Could you check a few things on this model? Use its own coordinates, in mm. A direction names the side the tool comes from. Coordinates: 2 decimals unless noted, no trailing zeros. Write each loop counter-clockwise with the first axis right and the second up, starting at its lowest first coordinate (ties: lowest second). Pieces come first, ordered by that corner, then holes.
```python
from build123d import *

# Parameters (mm, degrees)
EXTRUDE_1_DEPTH         = 3
SKETCH_2_W              = 1.5
SKETCH_2_H              = 5
CUT_EXTRUDE_1_DEPTH     = 154.658257181
SKETCH_3_W              = 54.5
SKETCH_3_H              = 3
EXTRUDE_2_DEPTH         = 40
HOLE_WIZARD_2_5_2_5_1_D = 2.5
HOLE_WIZARD_2_5_2_5_2_D = 2.5
HOLE_WIZARD_M641_D      = 71.5
FILLET_1_R              = 0.5
FILLET_2_R              = 3
FILLET_3_R              = 3.5
FILLET_4_R              = 44.4


with BuildPart() as part:
    # Эскиз1 → Бобышка-Вытянуть1 (new body)
    with BuildSketch(Plane.XZ.offset(-148.5)):
        with BuildLine():
            Line((121.9, -25.878684783), (121.9, 53.4))
            Line((121.9, 53.4), (-121.9, 53.4))
            Line((-121.9, 53.4), (-121.9, -25.878684783))
            ThreePointArc((-121.9, -25.878684783), (-115.016337378, -38.133733536), (-104.847515108, -47.837654634))
            Line((-104.847515108, -47.837654634), (-40, -93.5))
            Line((-40, -93.5), (39.841624635, -93.5))
            Line((39.841624635, -93.5), (39.841624635, -88.5))
            Line((39.841624635, -88.5), (41.341624635, -88.5))
            Line((41.341624635, -88.5), (41.341624635, -92.555295683))
            Line((41.341624635, -92.555295683), (104.847515108, -47.837654634))
            ThreePointArc((104.847515108, -47.837654634), (115.016337378, -38.133733536), (121.9, -25.878684783))
        make_face()
    extrude(amount=-EXTRUDE_1_DEPTH)

    # Эскиз2 → Вырез-Вытянуть1 (cut, through all)
    with BuildSketch(Plane(origin=(0, 151.5, 0), x_dir=(-1, 0, 0), z_dir=(0, 1, 0))):
        with Locations((15.408375365, -91)):
            Rectangle(SKETCH_2_W, SKETCH_2_H)
    extrude(amount=-CUT_EXTRUDE_1_DEPTH, mode=Mode.SUBTRACT)

    # Эскиз3 → Бобышка-Вытянуть2 (add)
    with BuildSketch(Plane.XZ.offset(-148.5)):
        with Locations((12.591624635, -92)):
            Rectangle(SKETCH_3_W, SKETCH_3_H)
    extrude(amount=EXTRUDE_2_DEPTH)

    # Диаметр отверстия Ø2.5 (2.5)1 (through all)
    with Locations(Plane(origin=(0, 148.5, 0), x_dir=(-1, 0, 0), z_dir=(0, -1, 0))):
        with Locations((40, 57.5), (40, 77.5), (20, 57.5), (20, 77.5), (-40, 57.5), (-40, 77.5), (-20, 57.5), (-20, 77.5), (0, 57.5), (0, 77.5)):
            Hole(HOLE_WIZARD_2_5_2_5_1_D / 2)

    # Диаметр отверстия Ø2.5 (2.5)2 (through all)
    with Locations(Plane.XY.offset(-90.5)):
        with Locations((25, 116.5), (25, 132.5), (0, 116.5), (0, 132.5)):
            Hole(HOLE_WIZARD_2_5_2_5_2_D / 2)

    # Отверстие с зазором M641 (through all)
    with Locations(Plane(origin=(0, 148.5, 0), x_dir=(-1, 0, 0), z_dir=(0, -1, 0))):
        with Locations((72, 0), (-72, 0)):
            Hole(HOLE_WIZARD_M641_D / 2)

    # Скругление1
    fillet_1_edges = [part.edges().sort_by_distance(p)[0] for p in [
        (-40, 150, -93.5),
        (12.591624635, 148.5, -90.5),
    ]]
    fillet(fillet_1_edges, radius=FILLET_1_R)

    # Скругление2
    fillet_2_edges = [part.edges().sort_by_distance(p)[0] for p in [
        (-14.658375365, 108.5, -92),
        (39.841624635, 108.5, -92),
    ]]
    fillet(fillet_2_edges, radius=FILLET_2_R)

    # Скругление3
    fillet_3_edges = [part.edges().sort_by_distance(p)[0] for p in [
        (12.591624635, 151.5, -93.5),
    ]]
    fillet(fillet_3_edges, radius=FILLET_3_R)

    # Скругление4
    fillet_4_edges = [part.edges().sort_by_distance(p)[0] for p in [
        (-121.9, 150, 53.4),
        (121.9, 150, 53.4),
    ]]
    fillet(fillet_4_edges, radius=FILLET_4_R)


solid = part.part
```
1. I want a section at D-D on z = -16.5. Please give me the cut outline in (x, y).
Verdict:
outline: (-121.9, 148.5) - (-103.71, 148.5) - (-103.71, 151.5) - (-121.9, 151.5) - close; (-40.29, 148.5) - (40.29, 148.5) - (40.29, 151.5) - (-40.29, 151.5) - close; (103.71, 148.5) - (121.9, 148.5) - (121.9, 151.5) - (103.71, 151.5) - close
2. On a 3-axis mill with a long thin cutter (end or side, diameter ignored), from which of +Z, -Z, +X, -X, +Y, -Y can I reach the whole of each face in a straight line? I mean faces 5 (the face through (-115.137, 149.979, -37.977)), 6 (the face through (12, 129, -90.5)), 7 (the face through (39.842, 132, -92)). Say none if no direction works.
Verdict:
face 5: -Z, -X, +Y, -Y
face 6: +Z, +X, -X, -Y
face 7: -Z, +Y, -Y
3. I want a section at C-C on y = 122. Please give me the cut outline in (x, z).
Verdict:
outline: (-14.66, -93.5) - (39.84, -93.5) - (39.84, -90.5) - (-14.66, -90.5) - close
4. If we mould it in two halves opening along X, with no side actions, what happens to faces 1 (the face through (72.65, 149.98, -70.51)), 2 (the face through (43.63, 150.021, 21.753)), 3 (the face through (-2, 148.5, -19)), 4 (the face through (-37.9, 150.02, -10.74))? For each: pulls with the +X half, pulls with the -X half, needs draft (parallel to the pull), parting line crosses it, or undercut.
Verdict:
face 1: pulls with the +X half
face 2: undercut
face 3: needs draft
face 4: undercut
5. For pin 1 (1.5 mm diameter, centred on x = -40, z = -77.5, fed in from -Y); pin 2 (6 mm diameter, centred on x = 91, z = 38.5, fed in from -Y); pin 3 (1.2 mm diameter, centred on x = 40.5, y = 149.5, fed in from -Z); pin 4 (3 mm diameter, centred on x = 20, z = -77.5, fed in from +Y), each with a flat end and sliding along its axis, tell me the tip position at first contact or that it passes through.
Verdict:
pin 1: passes through
pin 2: stops at y = 148.5
pin 3: stops at z = -88.5
pin 4: stops at y = 151.5
6. Please list where these lines run through material, in increasing order: line 1 along X through (y, z) = (150.35, -77.5); line 2 along Z through (x, y) = (0, 149.4); line 3 along Y through (x, z) = (0, -92.75).
Verdict:
line 1: x = -62.72 to -41.25, -38.75 to -21.25, -18.75 to -1.25, 1.25 to 18.75, 21.25 to 38.75, 41.25 to 62.72
line 2: z = -93.21 to -78.75, -76.25 to -58.75, -56.25 to 53.4
line 3: y = 108.5 to 115.25, 117.75 to 131.25, 133.75 to 150.17
7. I want a section at A-A on x = 9. Please give me the cut outline in (y, z), plus the area to 3 significant figures.
Verdict:
outline: (108.5, -93.5) - (148, -93.5) arc R3.5 ccw to (151.5, -90) - (151.5, 53.4) - (148.5, 53.4) - (148.5, -90) arc R0.5 cw to (148, -90.5) - (108.5, -90.5) - close
area: 558 mm2
8. I want a section at B-B on z = 28. Please give me the cut outline in (x, y), plus the area to 3 significant figures.
Verdict:
outline: (-117.63, 148.5) - (-94.23, 148.5) - (-94.23, 151.5) - (-117.63, 151.5) - close; (-49.77, 148.5) - (49.77, 148.5) - (49.77, 151.5) - (-49.77, 151.5) - close; (94.23, 148.5) - (117.63, 148.5) - (117.63, 151.5) - (94.23, 151.5) - close
area: 439 mm2
